from build123d import *

# Parameters (mm, degrees)
ESBO_O2_R                = 4.15
ESBO_O2_W                = 3
ESBO_O2_H                = 5.5
ESBO_O2_W_2              = 20
ESBO_O2_H_2              = 25
RESSALTO_EXTRUS_O1_DEPTH = 6
ESBO_O4_R                = 1.6
RESSALTO_EXTRUS_O2_DEPTH = 4
RESSALTO_EXTRUS_O3_START = 20
ESBO_O4_2_R              = 1.6
RESSALTO_EXTRUS_O3_DEPTH = 4
CORTE_EXTRUS_O2_START    = -1
ESBO_O7_R                = 1.65
CORTE_EXTRUS_O2_DEPTH    = 8.8
CORTE_EXTRUS_O3_START    = -1
ESBO_O8_R                = 1.65
CORTE_EXTRUS_O3_DEPTH    = 8.8


with BuildPart() as part:
    # Esboço2 → Ressalto-extrusão1 (new body)
    with BuildSketch(Plane(origin=(0, 0, 0), x_dir=(1, 0, 0), z_dir=(0, 1, 0))):
        with BuildLine():
            Line((-0.794404607, 46.121664503), (69.205595393, 51.121664503))
            ThreePointArc((69.205595393, 51.121664503), (77.59818691, 48.160273015), (81.15, 40))
            Line((81.15, 40), (81.15, 32.5))
            Line((81.15, 32.5), (51.15, 32.5))
            Line((51.15, 32.5), (51.15, -32.5))
            Line((51.15, -32.5), (81.15, -32.5))
            Line((81.15, -32.5), (81.15, -40))
            ThreePointArc((81.15, -40), (77.59818691, -48.160273015), (69.205595393, -51.121664503))
            Line((69.205595393, -51.121664503), (-0.794404607, -46.121664503))
            ThreePointArc((-0.794404607, -46.121664503), (-8.160273015, -42.59818691), (-11.15, -35))
            Line((-11.15, -35), (-11.15, 35))
            ThreePointArc((-11.15, 35), (-8.160273015, 42.59818691), (-0.794404607, 46.121664503))
        make_face()
        with Locations((0, 35)):
            Circle(ESBO_O2_R, mode=Mode.SUBTRACT)
        with Locations((70, 40)):
            Circle(ESBO_O2_R, mode=Mode.SUBTRACT)
        with Locations((70, -40)):
            Circle(ESBO_O2_R, mode=Mode.SUBTRACT)
        with Locations((0, -35)):
            Circle(ESBO_O2_R, mode=Mode.SUBTRACT)
        with Locations((-5.85, 35)):
            Rectangle(ESBO_O2_W, ESBO_O2_H, mode=Mode.SUBTRACT)
        with Locations((75.85, 40)):
            Rectangle(ESBO_O2_W, ESBO_O2_H, mode=Mode.SUBTRACT)
        with Locations((75.85, -40)):
            Rectangle(ESBO_O2_W, ESBO_O2_H, mode=Mode.SUBTRACT)
        with Locations((-5.85, -35)):
            Rectangle(ESBO_O2_W, ESBO_O2_H, mode=Mode.SUBTRACT)
        with Locations((21.15, 0)):
            Rectangle(ESBO_O2_W_2, ESBO_O2_H_2, mode=Mode.SUBTRACT)
    extrude(amount=RESSALTO_EXTRUS_O1_DEPTH)

    # Esboço4 → Ressalto-extrusão2 (add)
    with BuildSketch(Plane(origin=(11.15, 0, 0), x_dir=(0, 0, -1), z_dir=(1, 0, 0))):
        with BuildLine():
            Line((-4, -4), (-4, 0))
            Line((-4, 0), (4, 0))
            Line((4, 0), (4, -4))
            ThreePointArc((4, -4), (0, -8), (-4, -4))
        make_face()
        with Locations((0, -4)):
            Circle(ESBO_O4_R, mode=Mode.SUBTRACT)
    extrude(amount=-RESSALTO_EXTRUS_O2_DEPTH)

    # Esboço4<2> → Ressalto-extrusão3 (add)
    with BuildSketch(Plane(origin=(11.15, 0, 0), x_dir=(0, 0, -1), z_dir=(1, 0, 0)).offset(RESSALTO_EXTRUS_O3_START)):
        with BuildLine():
            Line((-4, -4), (-4, 0))
            Line((-4, 0), (4, 0))
            Line((4, 0), (4, -4))
            ThreePointArc((4, -4), (0, -8), (-4, -4))
        make_face()
        with Locations((0, -4)):
            Circle(ESBO_O4_2_R, mode=Mode.SUBTRACT)
    extrude(amount=RESSALTO_EXTRUS_O3_DEPTH)

    # Esboço7 → Corte-extrusão2 (cut)
    with BuildSketch(Plane(origin=(74.35, 0, 0), x_dir=(0, 0, -1), z_dir=(1, 0, 0)).offset(CORTE_EXTRUS_O2_START)):
        with Locations((40, 3)):
            Circle(ESBO_O7_R)
    corte_extrus_o2 = extrude(amount=CORTE_EXTRUS_O2_DEPTH, mode=Mode.SUBTRACT)

    # Esboço8 → Corte-extrusão3 (cut)
    with BuildSketch(Plane.ZY.offset(4.35).offset(CORTE_EXTRUS_O3_START)):
        with Locations((35, 3)):
            Circle(ESBO_O8_R)
    corte_extrus_o3 = extrude(amount=CORTE_EXTRUS_O3_DEPTH, mode=Mode.SUBTRACT)

    # Espelhar1: Corte-extrusão2, Corte-extrusão3 across plane
    add(corte_extrus_o2.mirror(Plane.XY), mode=Mode.SUBTRACT)
    add(corte_extrus_o3.mirror(Plane.XY), mode=Mode.SUBTRACT)


solid = part.part
Here's how the part is built. I have some questions about the finished solid (model axes, mm). A direction names the side the tool comes from. Coordinates: 2 decimals unless noted, no trailing zeros. Loops run counter-clockwise (first coordinate to the right, second up) from the corner with the lowest first, then second, coordinate; pieces in that order, holes last.
1. Imagine slicing it at A-A, the plane z = 0. Please give me the cut outline in (x, y).
2. I need wall thicknesses on L1, parallel to Y at x = 78.35, z = 40; L2, parallel to Z at x = -4.1, y = 3; L3, parallel to Z at x = -0.5, y = 2.75. Which ranges of each line are inside material? Lowest first, please.
3. Imagine slicing it at B-B, the plane x = 10. Please give me the cut outline in (y, z), and give its area (3 significant figures).
4. For P1, Ø3.5, axis at x = 76, y = 4, coming from the +Z side; P2, Ø3.5, axis at x = 75, y = 2, coming from the -Z side; P3, Ø0.9, axis at x = 76, y = 2.5, coming from the +Z side, each with a flat end and sliding along its axis, tell me the tip position at first contact or that it passes through.
5. For faces 5 (the cylindrical face through (-9.22, 3.07, -33.35)), 6 (the flat face through (66, 3, 32.5)), 7 (the flat face through (77.35, 1.6, -38.7)), which set-ups out of +Z, -Z, +X, -X, +Y, -Y let a thin tool reach every point of the face, with its end or its side?
6. If we mould it in two halves opening along X, with no side actions, what happens to faces 1 (the flat face through (-7.35, 1.6, 33.8)), 2 (the flat face through (66, 3, -32.5)), 3 (the cylindrical face through (3.834, 2.958, -33.411)), 4 (the flat face through (-11.15, 3, 0))? For each: pulls with the +X half, pulls with the -X half, needs draft (parallel to the pull), parting line crosses it, or undercut.
7. Imagine slicing it at C-C, the plane z = -25. Please give me the cut outline in (x, y), and give its area (3 significant figures).
Taken from the geometry:
1. outline: (-11.15, 0) - (7.15, 0) - (7.15, -2.4) - (11.15, -2.4) - (11.15, 6) - (-11.15, 6) - close; (7.15, -8) - (11.15, -8) - (11.15, -5.6) - (7.15, -5.6) - close; (31.15, -8) - (35.15, -8) - (35.15, -5.6) - (31.15, -5.6) - close; (31.15, -2.4) - (35.15, -2.4) - (35.15, 0) - (51.15, 0) - (51.15, 6) - (31.15, 6) - close
2. L1: y = 0 to 1.35, 4.65 to 6
2. L2: z = -45.37 to -36.65, -33.35 to 33.35, 36.65 to 45.37
2. L3: z = -46.14 to -39.12, -30.88 to 30.88, 39.12 to 46.14
3. outline: (-4, -4) - (0, -4) - (0, -46.89) - (6, -46.89) - (6, 46.89) - (0, 46.89) - (0, 4) - (-4, 4) arc R4 ccw to start; hole circle Ø3.2 at (-4, 0)
3. area: 612 mm2
4. P1: stops at z = 50.31
4. P2: stops at z = -50.67
4. P3: stops at z = 49.67
5. face 5: -X
5. face 6: +X, +Y, -Y
5. face 7: +Y, -Y
6. face 1: undercut
6. face 2: needs draft
6. face 3: undercut
6. face 4: pulls with the -X half
7. outline: (-11.15, 0) - (51.15, 0) - (51.15, 6) - (-11.15, 6) - close
7. area: 374 mm2
